Part model, mm, in its own coordinate system. Face numbers are marked on the shaded views. A direction names the side the tool comes from. Give positions to 0.01 mm unless a question says otherwise; leave off trailing zeros. Write each loop counter-clockwise with the first axis right and the second up, starting at its lowest first coordinate (ties: lowest second). Pieces come first, ordered by that corner, then holes. Notation, with made-up numbers: (-34, 58) - (22, 58) arc R21 ccw to (22, 83) - close; hole circle Ø1 at (45.5, -20.75). An arc over 180 degrees is marked (long way). Answer as a JSON object with one key per item and string values. Group by question number.
Autodesk Inventor part; units mm, degrees
ref_plane "YZ Plane" through (0, 0, 0) normal (1, 0, 0) x (0, 1, 0)
ref_plane "XZ Plane" through (0, 0, 0) normal (0, 1, 0) x (-1, 0, 0)
ref_plane "XY Plane" through (0, 0, 0) normal (0, 0, 1) x (1, 0, 0)
sketch "Sketch1" plane through (0, 0, 0) normal (0, 1, 0) x (-1, 0, 0)
  line L0 (0, 0) -> (101.6, 0)
  line L1 (101.6, 0) -> (101.6, -127)
  line L2 (101.6, -127) -> (0, -127)
  line L3 (0, -127) -> (0, 0)
  dimension "d0" = 101.6
  dimension "d1" = 127
extrude "Extrusion1" add sketch "Sketch1" along normal blind 6.35
sketch "Sketch2" plane through (0, 6.35, 0) normal (0, 1, 0) x (1, 0, 0)
  line L0 (-82.55, 5.08) -> (-25.4, 5.08)
  line L1 (-22.4915, 9.8367) -> (-22.4915, 13.0117)
  line L2 (-25.3966, 17.78) -> (-82.55, 17.78)
  line L3 (-82.55, 17.78) -> (-82.55, 5.08)
  arc A0 (-25.4, 5.08) -> (-22.4915, 9.8367) centre (-22.6493, 6.6656) ccw
  arc A1 (-22.4915, 13.0117) -> (-25.3966, 17.78) centre (-22.6527, 16.1826) ccw
  line L4 (-101.6, 127) -> (-101.6, 0)
  line L5 (-101.6, 0) -> (0, 0)
  line L6 (-82.55, 30.48) -> (-25.4, 30.48)
  line L7 (-22.4915, 35.2367) -> (-22.4915, 38.4117)
  line L8 (-25.3966, 43.18) -> (-82.55, 43.18)
  line L9 (-82.55, 43.18) -> (-82.55, 30.48)
  arc A2 (-25.4, 30.48) -> (-22.4915, 35.2367) centre (-22.6493, 32.0656) ccw
  arc A3 (-22.4915, 38.4117) -> (-25.3966, 43.18) centre (-22.6527, 41.5826) ccw
  line L10 (-82.55, 55.88) -> (-25.4, 55.88)
  line L11 (-22.4915, 60.6367) -> (-22.4915, 63.8117)
  line L12 (-25.3966, 68.58) -> (-82.55, 68.58)
  line L13 (-82.55, 68.58) -> (-82.55, 55.88)
  arc A4 (-25.4, 55.88) -> (-22.4915, 60.6367) centre (-22.6493, 57.4656) ccw
  arc A5 (-22.4915, 63.8117) -> (-25.3966, 68.58) centre (-22.6527, 66.9826) ccw
  line L14 (-82.55, 81.28) -> (-25.4, 81.28)
  line L15 (-22.4915, 86.0367) -> (-22.4915, 89.2117)
  line L16 (-25.3966, 93.98) -> (-82.55, 93.98)
  line L17 (-82.55, 93.98) -> (-82.55, 81.28)
  arc A6 (-25.4, 81.28) -> (-22.4915, 86.0367) centre (-22.6493, 82.8656) ccw
  arc A7 (-22.4915, 89.2117) -> (-25.3966, 93.98) centre (-22.6527, 92.3826) ccw
  line L18 (-82.55, 106.68) -> (-25.4, 106.68)
  line L19 (-22.4915, 111.4367) -> (-22.4915, 114.6117)
  line L20 (-25.3966, 119.38) -> (-82.55, 119.38)
  line L21 (-82.55, 119.38) -> (-82.55, 106.68)
  arc A8 (-25.4, 106.68) -> (-22.4915, 111.4367) centre (-22.6493, 108.2656) ccw
  arc A9 (-22.4915, 114.6117) -> (-25.3966, 119.38) centre (-22.6527, 117.7826) ccw
  point P0 (-82.55, 11.43)
  point P1 (-82.55, 36.83)
  point P2 (-82.55, 62.23)
  point P3 (-82.55, 87.63)
  point P4 (-82.55, 113.03)
  dimension "d5" = 12.7
  dimension "d6" = 6.35
  dimension "d7" = 6.35
  dimension "d8" = 3.175
  dimension "d9" = 57.15
  dimension "d10" = 19.05
  dimension "d11" = 5.08
  dimension "d14" = 25.4
extrude "Extrusion2" cut sketch "Sketch2" against normal blind 2.921
properties part number "mold plate with alignment"
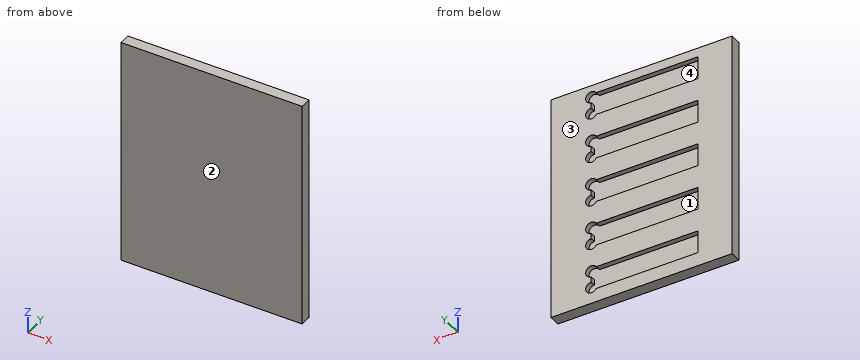
1) Saw through at A-A (y = 5). State how many separate pieces and enclosed holes the cut face has, and give its area (3 significant figures).
2) Drill centre lines: line 1 along Z through (x, y) = (-80, 3.5); line 2 along X through (y, z) = (3.75, -10.5); line 3 along Y through (x, z) = (-64, -82.5). Where is each one in solid material? Low to high. Write a range as from..to.
3) Drop a flat-ended pin along its axis: P1, Ø5.5, axis at x = -22.65, z = -6.67, coming from the +Y side. Give the stop position or say it passes through.
4) Saw through at B-B (x = -27). List the corners of the cut face in (y, z), and give its area (3 significant figures).
5) Saw through at C-C (z = -118). List the corners of the cut face in (x, y), and give its area (3 significant figures).
6) Which spindle directions (+Z, -Z, +X, -X, +Y, -Y) get a long thin tool onto all of the face, cutting with end or side? Do the marked faces 1 and 2. Say none if no direction does.
7) Two-plate mould, pull along X, no slides. Class the marked faces 3 and 4: +X half, -X half, draft (parallel to the pull), parting line (faces both ways), or undercut.
Checks:
{
 "1": {"separate pieces": "1", "enclosed holes": "5", "area": "8,910 mm2"},
 "2": {"line 1": "-127..-119.38, -106.68..-93.98, -81.28..-68.58, -55.88..-43.18, -30.48..-17.78, -5.08..0", "line 2": "-101.6..-82.55, -22.49..0", "line 3": "0..3.43"},
 "3": {"P1": "y = 3.43"},
 "4": {"outline": "(0, -127) - (6.35, -127) - (6.35, -119.38) - (3.43, -119.38) - (3.43, -106.68) - (6.35, -106.68) - (6.35, -93.98) - (3.43, -93.98) - (3.43, -81.28) - (6.35, -81.28) - (6.35, -68.58) - (3.43, -68.58) - (3.43, -55.88) - (6.35, -55.88) - (6.35, -43.18) - (3.43, -43.18) - (3.43, -30.48) - (6.35, -30.48) - (6.35, -17.78) - (3.43, -17.78) - (3.43, -5.08) - (6.35, -5.08) - (6.35, 0) - (0, 0) - close", "area": "621 mm2"},
 "5": {"outline": "(-101.6, 0) - (0, 0) - (0, 6.35) - (-19.49, 6.35) - (-19.49, 3.43) - (-82.55, 3.43) - (-82.55, 6.35) - (-101.6, 6.35) - close", "area": "461 mm2"},
 "6": {"face 1": "+Y", "face 2": "+Z, -Z, +X, -X, -Y"},
 "7": {"face 3": "draft", "face 4": "undercut"}
}
